For this review, use the dimensioned drawing (mm, ordinates from the lowest corner) and the shaded views. A direction names the side the tool comes from. Coordinates: 2 decimals unless noted, no trailing zeros. Order: outer loops, then holes, each group sorted by start corner. A loop starts at its lowest first (then second) coordinate and runs counter-clockwise, first axis right, second up. Notation, with made-up numbers: M 58.5,24 L 85.5,24 A9 cw 85.5,37 Z; hole C 73.25,35 d1. An arc over 180 degrees is marked long. Write each question's results on one line, items separated by ' | '.
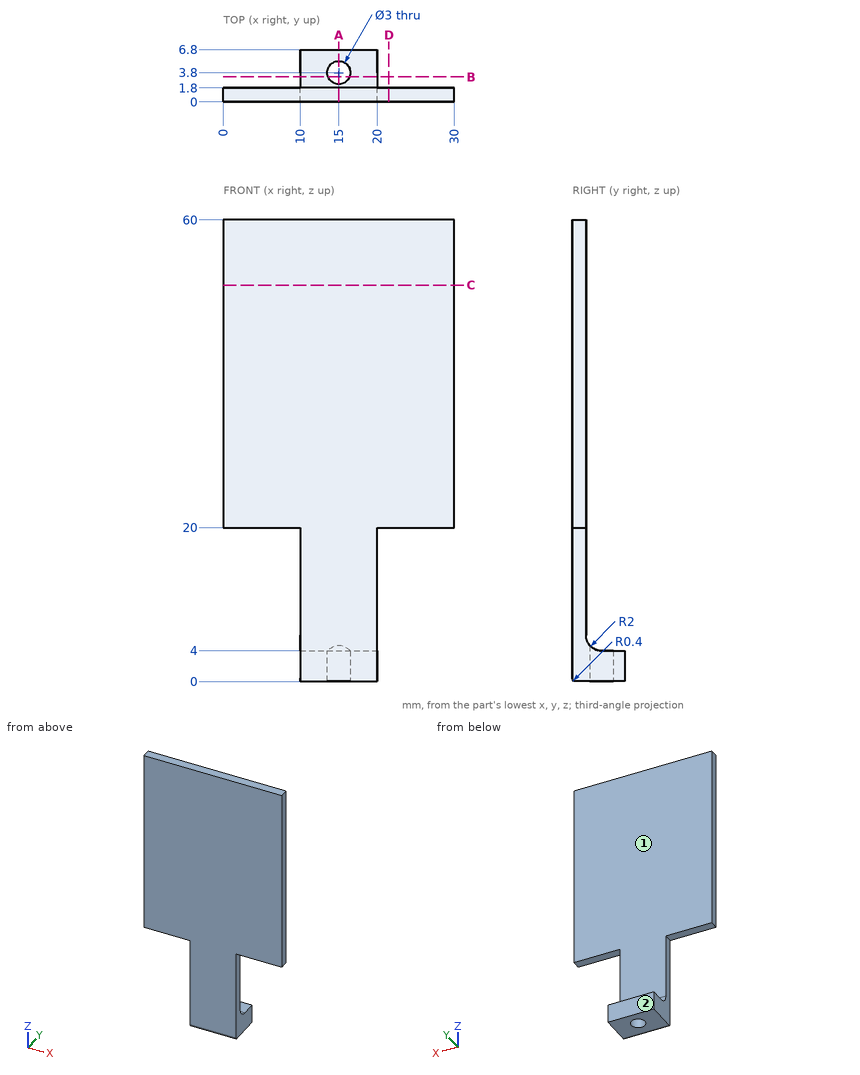
1) For the marked faces 1 and 2, list the 3-axis set-ups (+Z, -Z, +X, -X, +Y, -Y) from which the entire face can be reached by the end or side of a thin tool; tool diameter is ignored.
Solutions:
face 1: +Z, +X, -X, +Y | face 2: +Z, -Z, +X, -X, +Y
2) To check wall thickness, follow line 1 along Y through (x, z) = (15, 3.15); line 2 along X through (y, z) = (3.8, 2); line 3 along Z through (x, y) = (7.5, 1.5). State the ranges of each line that lie inside material, in increasing order.
Solutions:
line 1: 0 to 2.3, 5.3 to 6.8 | line 2: 10 to 13.5, 16.5 to 20 | line 3: 20 to 60
3) For pin 1 (2.5 mm diameter, centred on x = 12.5, y = 6, fed in from +Z); pin 2 (6 mm diameter, centred on x = 12.5, z = 9.5, fed in from +Y); pin 3 (0.5 mm diameter, centred on x = 3.5, y = 1, fed in from -Z); pin 4 (2 mm diameter, centred on y = 4, z = 13.5, fed in from -X) (3 decimals), all flat-tipped, find the tip position at first contact; note any pin that passes through.
Solutions:
pin 1: z = 4 | pin 2: y = 1.8 | pin 3: z = 20 | pin 4: through
4) Take a section at A-A on x = 15. State the section outline as (y, z) points, plus the area to 3 significant figures.
Solutions:
outline: M 0,0.4 A0.4 ccw 0.4,0 L 2.3,0 L 2.3,4.68 A2 cw 1.8,6 L 1.8,60 L 0,60 Z; M 5.3,0 L 6.8,0 L 6.8,4 L 5.3,4 Z | area: 117 mm2
5) Take a section at D-D on x = 21.5. State the section outline as (y, z) points.
Solutions:
outline: M 0,20 L 1.8,20 L 1.8,60 L 0,60 Z
6) Take a section at B-B on y = 3.25. State the section outline as (x, z) points, plus the area to 3 significant figures.
Solutions:
outline: M 10,0 L 13.6,0 L 13.6,4.08 L 10,4.08 Z; M 16.4,0 L 20,0 L 20,4.08 L 16.4,4.08 Z | area: 29.4 mm2
7) Take a section at C-C on z = 51.5. State the section outline as (x, y) points, plus the area to 3 significant figures.
Solutions:
outline: M 0,0 L 30,0 L 30,1.8 L 0,1.8 Z | area: 54.0 mm2
